```python
from build123d import *


with BuildPart() as part:
    # Sketch1 → Revolve1 (revolve)
    with BuildSketch(Plane(origin=(0, 0, 0), x_dir=(0, 0, -1), z_dir=(1, 0, 0)), mode=Mode.PRIVATE) as revolve1_sk:
        Polygon((2, 5.8), (1.2, 5.8), (1.2, 5), (-1.8, 5), (-2, 4.8), (-2, 4.013736264), (-1.9, 4.013736264), (-1.9, 3.486263736), (-2, 3.486263736), (-2, 2.7), (-1.8, 2.5), (1.8, 2.5), (2, 2.7), (2, 3.486263736), (1.9, 3.486263736), (1.9, 4.013736264), (2, 4.013736264), align=None)
        with BuildLine():
            Line((-0.888888889, 4.013736264), (-0.927189449, 4.013736264))
            Line((-0.927189449, 4.013736264), (-0.927189449, 3.486263736))
            Line((-0.927189449, 3.486263736), (-0.888888889, 3.486263736))
            ThreePointArc((-0.888888889, 3.486263736), (0, 2.822810552), (0.888888889, 3.486263736))
            Line((0.888888889, 3.486263736), (0.927189449, 3.486263736))
            Line((0.927189449, 3.486263736), (0.927189449, 4.013736264))
            Line((0.927189449, 4.013736264), (0.888888889, 4.013736264))
            ThreePointArc((0.888888889, 4.013736264), (0, 4.677189449), (-0.888888889, 4.013736264))
        make_face(mode=Mode.SUBTRACT)
    revolve(revolve1_sk.sketch.rotate(Axis((0, 0, 0), (0, 0, 1)), 90), axis=Axis((0, 0, 0), (0, 0, 1)))


solid = part.part
```
CAD build for the part. Positions are in the model's coordinates, mm. A direction names the side the tool comes from. Give positions to 0.01 mm unless a question says otherwise; leave off trailing zeros. Loops run counter-clockwise (first coordinate to the right, second up) from the corner with the lowest first, then second, coordinate; pieces in that order, holes last. Notation, with made-up numbers: (-11.5, 4) -> (40.5, 4) arc R23 cw to (40.5, 34) -> close; hole circle Ø8 at (45, 60.5). An arc over 180 degrees is marked (long way). Use a Markdown table: item, result.
1. Which spindle directions (+Z, -Z, +X, -X, +Y, -Y) get a long thin tool onto all of the face, cutting with end or side? Do faces 1 (the flat face through (-0.6, -3.6, -1.9)), 2 (the flat face through (-2, -5, -1.2)), 3 (the flat face through (1, 3, -2)). Say none if no direction does.
Check result:
| item | result |
|---|---|
| face 1 | -Z |
| face 2 | +Z |
| face 3 | -Z, +X, -X, +Y, -Y |
2. Flat gauge pins, fed straight in: pin 1 (2.5 mm diameter, centred on x = 1.5, y = -1.5, fed in from +Z); pin 2 (2 mm diameter, centred on x = -3, z = 1.5, fed in from +Y). Where does each tip first touch, or does it go through?
Check result:
| item | result |
|---|---|
| pin 1 | stops at z = 2 |
| pin 2 | stops at y = 4.58 |
3. Mould opens along Z. For faces 4 (the flat face through (-1.37, -3.95, -2)), 5 (the cylindrical face through (5.794, -0.255, -1.594)), 6 (the flat face through (0.6, -3.6, 0.927)), 7 (the flat face through (3, 3, 2)) say: pulls with the +Z half, pulls with the -Z half, needs draft (parallel to the pull), parting line crosses it, or undercut.
Check result:
| item | result |
|---|---|
| face 4 | pulls with the -Z half |
| face 5 | needs draft |
| face 6 | undercut |
| face 7 | pulls with the +Z half |
4. Wall check: L1, parallel to Y at x = 0, z = -1.3; L2, parallel to Y at x = -1.25, z = -0.3; L3, parallel to Y at x = 0, z = -1.95. Give the ranges that are in metal, low to high. Write a range as [from, to].
Check result:
| item | result |
|---|---|
| L1 | y = [-5.8, -2.5], [2.5, 5.8] |
| L2 | y = [-4.84, -4.46], [-2.59, -2.17], [2.17, 2.59], [4.46, 4.84] |
| L3 | y = [-5.8, -4.01], [-3.49, -2.65], [2.65, 3.49], [4.01, 5.8] |
5. Slice it at C-C (z = 0.2). List the corners of the cut face in (x, y).
Check result:
| item | result |
|---|---|
| outline | circle Ø10 at (0, 0); circle Ø5.69 at (0, 0); hole circle Ø9.31 at (0, 0); hole circle Ø5 at (0, 0) |
6. Slice it at D-D (z = 1.6). List the corners of the cut face in (x, y), plus the area to 3 significant figures.
Check result:
| item | result |
|---|---|
| outline | circle Ø10 at (0, 0); hole circle Ø5 at (0, 0) |
| area | 58.9 mm^2 |
7. Slice it at A-A (y = 0). Give the number of separate pieces and of enclosed holes in the cut face, plus the area to 3 significant figures.
Check result:
| item | result |
|---|---|
| separate pieces | 2 |
| enclosed holes | 2 |
| area | 15.5 mm^2 |
